from build123d import *

# Parameters (mm, degrees)
SKICA1_W                 = 46
SKICA1_H                 = 20
P_IDAT_VYSUNUT_M1_DEPTH  = 2
SKICA2_W                 = 24
SKICA2_H                 = 13
ODEBRAT_VYSUNUT_M1_DEPTH = 2
SKICA3_R                 = 1
ODEBRAT_VYSUNUT_M2_DEPTH = 2


with BuildPart() as part:
    # Skica1 → Přidat vysunutím1 (new body)
    with BuildSketch(Plane(origin=(0, 0, 0), x_dir=(1, 0, 0), z_dir=(0, 1, 0))):
        Rectangle(SKICA1_W, SKICA1_H)
    extrude(amount=P_IDAT_VYSUNUT_M1_DEPTH)

    # Skica2 → Odebrat vysunutím1 (cut)
    with BuildSketch(Plane(origin=(0, 2, 0), x_dir=(1, 0, 0), z_dir=(0, 1, 0))):
        with Locations((-5.5, 0)):
            Rectangle(SKICA2_W, SKICA2_H)
    extrude(amount=-ODEBRAT_VYSUNUT_M1_DEPTH, mode=Mode.SUBTRACT)

    # Skica3 → Odebrat vysunutím2 (cut)
    with BuildSketch(Plane(origin=(0, 2, 0), x_dir=(1, 0, 0), z_dir=(0, 1, 0))):
        with Locations((-19.25, 0)):
            Circle(SKICA3_R)
        with Locations((8.25, 0)):
            Circle(SKICA3_R)
    extrude(amount=-ODEBRAT_VYSUNUT_M2_DEPTH, mode=Mode.SUBTRACT)


solid = part.part
Part model, mm, in its own coordinate system. A direction names the side the tool comes from. Coordinates: 2 decimals unless noted, no trailing zeros. Order: outer loops, then holes, each group sorted by start corner. A loop starts at its lowest first (then second) coordinate and runs counter-clockwise, first axis right, second up. Notation, with made-up numbers: M 57.5,72 L 90.5,72 A16 cw 90.5,89 Z; hole C 55.25,58 d2. An arc over 180 degrees is marked long. One line per question, with ' | ' between items.
Q1. 3-axis set-ups, long thin cutter, end or side, ignore diameter. For faces 1 (the face through (0, 2, -7)), 2 (the face through (-6, 1, 6.5)): which of +Z, -Z, +X, -X, +Y, -Y reach the whole face in a straight line?
A:
face 1: +Z, -Z, +X, -X, +Y | face 2: +Y, -Y
Q2. Slice it at B-B (x = 8.25). Give the cut face in (y, z), and give its area (3 significant figures).
A:
outline: M 0,-10 L 2,-10 L 2,-1 L 0,-1 Z; M 0,1 L 2,1 L 2,10 L 0,10 Z | area: 36.0 mm^2
Q3. Slice it at C-C (z = 3.25). Give the cut face in (x, y).
A:
outline: M -23,0 L -17.5,0 L -17.5,2 L -23,2 Z; M 6.5,0 L 23,0 L 23,2 L 6.5,2 Z
Q4. Slice it at D-D (z = 0). Give the cut face in (x, y).
A:
outline: M -23,0 L -20.25,0 L -20.25,2 L -23,2 Z; M -18.25,0 L -17.5,0 L -17.5,2 L -18.25,2 Z; M 6.5,0 L 7.25,0 L 7.25,2 L 6.5,2 Z; M 9.25,0 L 23,0 L 23,2 L 9.25,2 Z
Q5. Two-plate mould, pull along Z, no slides. Class faces 3 (the face through (23, 1, 0)), 4 (the face through (7.46, 1.01, 0.61)), 5 (the face through (0, 1, -10)): +Z half, -Z half, draft (parallel to the pull), parting line (faces both ways), or undercut.
A:
face 3: draft | face 4: undercut | face 5: -Z half
Q6. Drill centre lines: line 1 (X direction, y = 1.2, z = 0); line 2 (Z direction, x = 3, y = 0.3); line 3 (Z direction, x = 8.25, y = 0.85). Where is each one in solid material? Low to high.
A:
line 1: x = -23 to -20.25, -18.25 to -17.5, 6.5 to 7.25, 9.25 to 23 | line 2: z = -10 to -6.5, 6.5 to 10 | line 3: z = -10 to -1, 1 to 10
Q7. Slice it at A-A (y = 1.05). Give the cut face in (x, z), and give its area (3 significant figures).
A:
outline: M -23,-10 L 23,-10 L 23,10 L -23,10 Z; hole C -19.25,0 d2; hole M -17.5,-6.5 L 6.5,-6.5 L 6.5,6.5 L -17.5,6.5 Z; hole C 8.25,0 d2 | area: 602 mm^2
Q8. Pin check, flat tip, straight feed: P1, Ø2, axis at x = -1.5, z = -4, coming from the +Y side. Stop position of the tip, or through.
A:
P1: passes through
